from build123d import *

# Parameters (mm, degrees)
BASE_EXTRUDE_THIN_DEPTH = 800.1
SKETCH2_R               = 12.7
CUT_EXTRUDE1_DEPTH      = 815.930438749
LPATTERN1_COUNT         = 7
LPATTERN1_PITCH         = 107.95
BOSS_EXTRUDE1_START     = 38.1
BOSS_EXTRUDE1_OUTLINE_R = 9.525
BOSS_EXTRUDE1_DEPTH     = 19.05


# Read off the part's stored shape, not the designer's step: Boss-Extrude1
with BuildPart() as part:
    # Sketch1 → Base-Extrude-Thin (new body)
    with BuildSketch(Plane(origin=(0, 0, 0), x_dir=(0, 0, -1), z_dir=(1, 0, 0))):
        Polygon((-38.1, 0), (0, 0), (0, -150), (-38.1, -150), (-38.1, -146.825), (-3.175, -146.825), (-3.175, -3.175), (-38.1, -3.175), align=None)
    extrude(amount=BASE_EXTRUDE_THIN_DEPTH)

    # Sketch2 → Cut-Extrude1 (cut, through all)
    with BuildSketch(Plane(origin=(0, 0, 0), x_dir=(-1, 0, 0), z_dir=(0, 0, -1))):
        with Locations(Location((-50.8, -31.75, 0), (0, 0, 90))):
            Circle(SKETCH2_R)
    cut_extrude1 = extrude(amount=-CUT_EXTRUDE1_DEPTH, mode=Mode.SUBTRACT)

    # LPattern1: Cut-Extrude1 ×7
    with Locations(*[(i * LPATTERN1_PITCH, 0, 0) for i in range(1, LPATTERN1_COUNT)]):
        add(cut_extrude1, mode=Mode.SUBTRACT)

    # Boss-Extrude1 outline → Boss-Extrude1 (add)
    with BuildSketch(Plane.XY.offset(BOSS_EXTRUDE1_START)):
        with BuildLine():
            Line((101.6, 0), (101.6, -200))
            ThreePointArc((101.6, -200), (120.65, -219.05), (139.7, -200))
            Line((139.7, -200), (139.7, 0))
            Line((139.7, 0), (101.6, 0))
        make_face()
        with Locations((120.65, -200)):
            Circle(BOSS_EXTRUDE1_OUTLINE_R, mode=Mode.SUBTRACT)
    extrude(amount=BOSS_EXTRUDE1_DEPTH)


solid = part.part
For this review, take the finished solid that the model builds, in its own axes (mm). A direction names the side the tool comes from. Give positions to 0.01 mm unless a question says otherwise; leave off trailing zeros. Loops run counter-clockwise (first coordinate to the right, second up) from the corner with the lowest first, then second, coordinate; pieces in that order, holes last.
Item 1: Take a section at D-D, the plane y = -31.75. Give the number of separate pieces and of enclosed holes in the cut face, and give its area (3 significant figures).
Item 2: Tool access review of faces 5 (the flat face through (120, -74, 38.1)), 6 (the flat face through (139.7, -101, 47)), 7 (the flat face through (101.6, -99, 47)), 8 (the flat face through (406, 0, 22)): name each direction out of +Z, -Z, +X, -X, +Y, -Y from which nothing blocks a thin tool from reaching the whole face with its end or side.
Item 3: Draft analysis for pull direction X (two halves, no side actions). For faces 1 (the cylindrical face through (120.231, -219.045, 47.492)), 2 (the cylindrical face through (470.2, -34.5, 1.6)), 3 (the flat face through (800.1, -75, 2)), 4 (the flat face through (120, -108, 57.15)), state which applies: +X half, -X half, draft (parallel to the pull), parting line (faces both ways), or undercut.
Item 4: Take a section at C-C, the plane y = -110. State the section outline as (x, z) points (3 decimals), and give its area (3 significant figures).
Item 5: For line 1 along Y through (x, z) = (158, 2); line 2 along Y through (x, z) = (281, 34) (3 decimals); line 3 along Z through (x, y) = (292.5, -9) (3 decimals), list the stretches that pass through material, from the lowest coordinate up.
Item 6: Take a section at B-B, the plane z = 19.5. State the section outline as (x, y) points (3 decimals), and give its area (3 significant figures).
Item 7: Take a section at A-A, the plane x = 158.75. State the section outline as (y, z) points (3 decimals).
Item 8: Insertion check: pin 1 (2 mm diameter, centred on x = 358, y = -80.5, fed in from +Z) (3 decimals); pin 2 (1.5 mm diameter, centred on x = 456.5, z = 20.5, fed in from -Y); pin 3 (21 mm diameter, centred on y = -92, z = 44.5, fed in from -X). Each pin has a flat end and moves straight along its axis. Give the tip position at first contact, or say it passes through.
Calculated:
1. separate pieces: 9
1. enclosed holes: 0
1. area: 2,700 mm2
2. face 5: +X, -X
2. face 6: +Z, +X, +Y, -Y
2. face 7: +Z, -X, +Y, -Y
2. face 8: +Z, -Z, +X, -X, +Y
3. face 1: parting line
3. face 2: undercut
3. face 3: +X half
3. face 4: draft
4. outline: (0, 0) - (800.1, 0) - (800.1, 3.175) - (0, 3.175) - close; (101.6, 38.1) - (139.7, 38.1) - (139.7, 57.15) - (101.6, 57.15) - close
4. area: 3,270 mm2
5. line 1: y = -150 to -44.43, -19.07 to 0
5. line 2: y = -150 to -146.825, -3.175 to 0
5. line 3: z = 0 to 3.175
6. outline: (0, -150) - (800.1, -150) - (800.1, -146.825) - (0, -146.825) - close; (0, -3.175) - (800.1, -3.175) - (800.1, 0) - (0, 0) - close
6. area: 5,080 mm2
7. outline: (-150, 0) - (-44.45, 0) - (-44.45, 3.175) - (-146.825, 3.175) - (-146.825, 38.1) - (-150, 38.1) - close; (-19.05, 0) - (0, 0) - (0, 38.1) - (-3.175, 38.1) - (-3.175, 3.175) - (-19.05, 3.175) - close
8. pin 1: stops at z = 3.175
8. pin 2: stops at y = -150
8. pin 3: stops at x = 101.6
